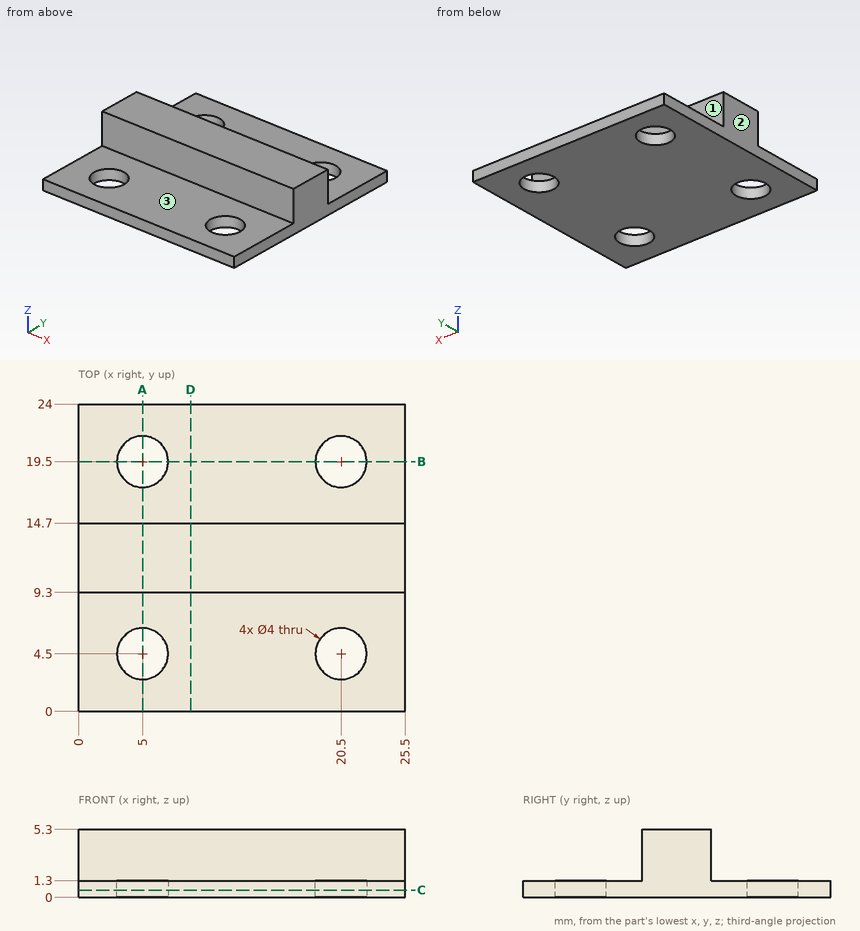
Check sheet for the drawn part. Datum: minimum x, y, z corner. Units: mm. A direction names the side the tool comes from. Round coordinates to 2 decimals unless told otherwise and drop trailing zeros. Order: outer loops, then holes, each group sorted by start corner. A loop starts at its lowest first (then second) coordinate and runs counter-clockwise, first axis right, second up. Notation, with made-up numbers: (3, 58.25) - (56, 58.25) arc R26 ccw to (56, 84.25) - close; hole circle Ø1 at (-13, 31). An arc over 180 degrees is marked (long way). Use a Markdown table: item, result. Add a question column.
(1) Material ranges on line 1 along Y through (x, z) = (5, 0.7); line 2 along Z through (x, y) = (1, 22.5); line 3 along Y through (x, z) = (10, 4.9), recorded low to high. Write a range as [from, to].
(2) Sectioned sample at A-A, the plane x = 5. Enter the section's corners in (y, z), and give its area (3 significant figures).
(3) Sectioned sample at C-C, the plane z = 0.55. Enter the section's corners in (x, y), and give its area (3 significant figures).
(4) Sectioned sample at B-B, the plane y = 19.5. Enter the section's corners in (x, z), and give its area (4 significant figures).
(5) Tool access check on the marked faces 1, 2 and 3. Record the directions out of +Z, -Z, +X, -X, +Y, -Y that give a thin tool (end or side, any length) a straight path to the whole face; none if there is none.
(6) Sectioned sample at D-D, the plane x = 8.75. Enter the section's corners in (y, z).
(7) Depth check by flat-ended pin: pin 1 (3 mm diameter, centred on x = 11, y = 19.5, fed in from +Z); pin 2 (2 mm diameter, centred on x = 9.5, z = 4, fed in from -Y). Enter the tip coordinate at first touch or a pass-through.
Answers below:
| question | item | result |
|---|---|---|
| 1 | line 1 | [0, 2.5], [6.5, 17.5], [21.5, 24] |
| 1 | line 2 | [0, 1.3] |
| 1 | line 3 | [9.3, 14.7] |
| 2 | outline | (0, 0) - (2.5, 0) - (2.5, 1.3) - (0, 1.3) - close; (6.5, 0) - (17.5, 0) - (17.5, 1.3) - (14.7, 1.3) - (14.7, 5.3) - (9.3, 5.3) - (9.3, 1.3) - (6.5, 1.3) - close; (21.5, 0) - (24, 0) - (24, 1.3) - (21.5, 1.3) - close |
| 2 | area | 42.4 mm² |
| 3 | outline | (0, 0) - (25.5, 0) - (25.5, 24) - (0, 24) - close; hole circle Ø4 at (5, 4.5); hole circle Ø4 at (5, 19.5); hole circle Ø4 at (20.5, 4.5); hole circle Ø4 at (20.5, 19.5) |
| 3 | area | 562 mm² |
| 4 | outline | (0, 0) - (3, 0) - (3, 1.3) - (0, 1.3) - close; (7, 0) - (18.5, 0) - (18.5, 1.3) - (7, 1.3) - close; (22.5, 0) - (25.5, 0) - (25.5, 1.3) - (22.5, 1.3) - close |
| 4 | area | 22.75 mm² |
| 5 | face 1 | +Z, +X, -X, +Y |
| 5 | face 2 | +Z, -Z, -X, +Y, -Y |
| 5 | face 3 | +Z, +X, -X, -Y |
| 6 | outline | (0, 0) - (24, 0) - (24, 1.3) - (14.7, 1.3) - (14.7, 5.3) - (9.3, 5.3) - (9.3, 1.3) - (0, 1.3) - close |
| 7 | pin 1 | z = 1.3 |
| 7 | pin 2 | y = 9.3 |
